Job drawing, mm, ordinate dimensions from the low corner. One solid piece. Coordinates: 2 decimals unless noted, no trailing zeros. Loops run counter-clockwise (first coordinate to the right, second up) from the corner with the lowest first, then second, coordinate; pieces in that order, holes last. Notation, with made-up numbers: (37.5, 24.25) - (61.5, 24.25) arc R18 ccw to (61.5, 45.25) - close; hole circle Ø4 at (-23, 42). An arc over 180 degrees is marked (long way). Use a Markdown table: item, result. Add a question column.
1) Band-saw the part on A-A (y = 79). Give the cut face in (x, z).
2) Probe probe 1 along Y at (x, z) = (79, 106); probe 2 along X at (y, z) = (105, 14); probe 3 along X at (y, z) = (108.5, 82). List the from-to ranges inside material, lowest first. Write a range as [from, to].
3) Pull direction Y, two halves, no side cores. Call the marked faces 1 and 2: +Y half, -Y half, draft (parallel to the pull), parting line (faces both ways), or undercut.
4) Band-saw the part on C-C (z = 92). Give the cut face in (x, y).
5) Drop flat-ended pins along their axis: P1, Ø3, axis at x = 60.5, z = 42, coming from the +Y side; P2, Ø4, axis at x = 135, z = 133.5, coming from the -Y side. Give the stop position or say it passes through.
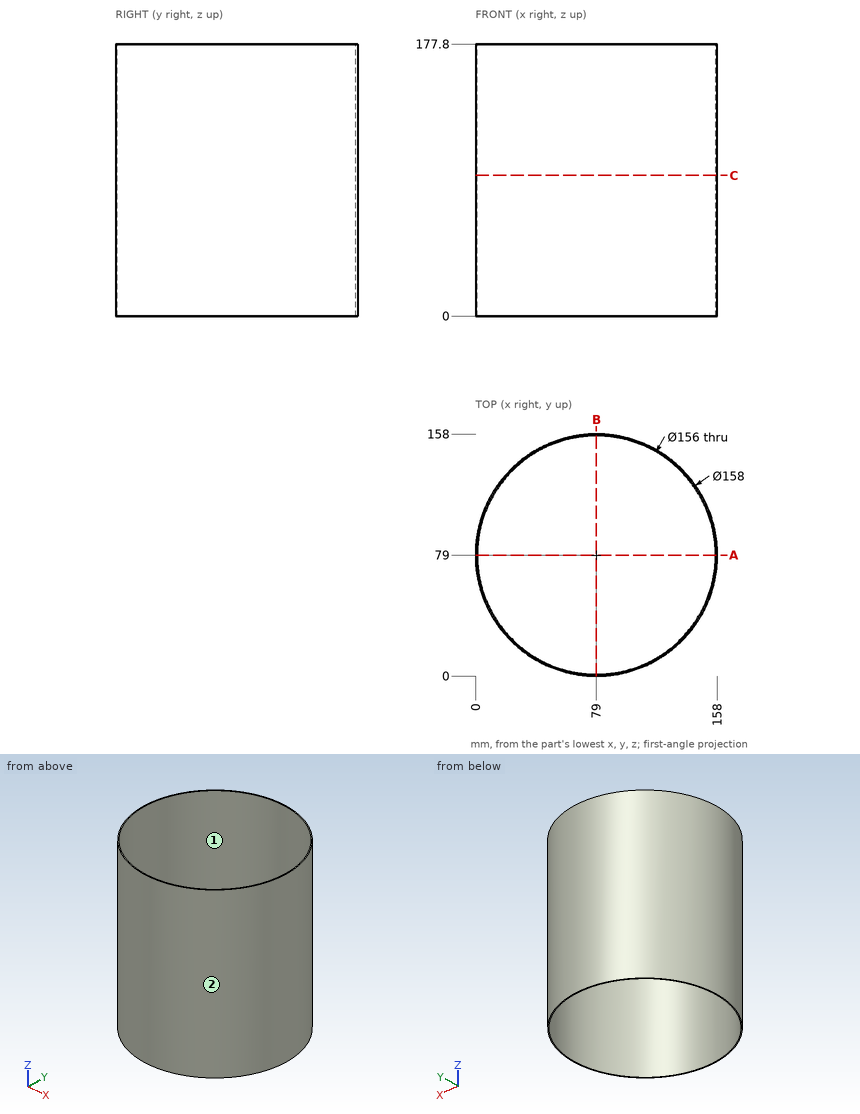
Answer block:
| question | item | result |
|---|---|---|
| 1 | outline | (0, 0) - (1, 0) - (1, 177.8) - (0, 177.8) - close; (157, 0) - (158, 0) - (158, 177.8) - (157, 177.8) - close |
| 2 | probe 1 | [0, 1], [157, 158] |
| 2 | probe 2 | [4.4, 5.46], [152.54, 153.6] |
| 2 | probe 3 | [5.71, 6.79], [151.21, 152.29] |
| 3 | face 1 | undercut |
| 3 | face 2 | parting line |
| 4 | outline | circle Ø158 at (79, 79); hole circle Ø156 at (79, 79) |
| 5 | P1 | y = 156.15 |
| 5 | P2 | y = 21.34 |
